Geometry check sheet. Reference: the model listing, model coordinates, mm. Face numbers are marked on the shaded views. A direction names the side the tool comes from. Coordinates: 2 decimals unless noted, no trailing zeros. Write each loop counter-clockwise with the first axis right and the second up, starting at its lowest first coordinate (ties: lowest second). Pieces come first, ordered by that corner, then holes.
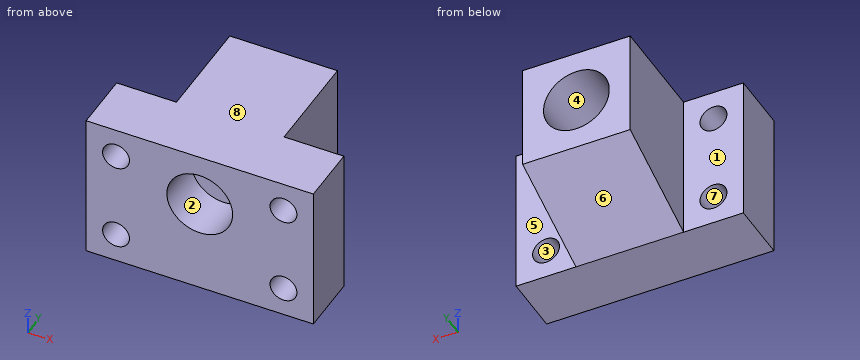
from build123d import *

# Parameters (mm, degrees)
SALIENTE_EXTRUIR1_DEPTH      = 18
SALIENTE_EXTRUIR1_DEPTH_BACK = 32
CROQUIS2_R                   = 11
CORTAR_EXTRUIR1_DEPTH        = 30
CORTAR_EXTRUIR2_START        = -16
CROQUIS3_R                   = 11
CORTAR_EXTRUIR2_DEPTH        = 16
CORTAR_EXTRUIR3_REACH        = 60.034
CROQUIS4_R                   = 5.5
CORTAR_EXTRUIR4_REACH        = 86.764
CORTAR_EXTRUIR5_REACH        = 62.77
CROQUIS6_R                   = 4.5


with BuildPart() as part:
    # Croquis1 → Saliente-Extruir1 (new, two sides: drawn at the far end of the back side and taken through both)
    with BuildSketch(Plane.XY.offset(-SALIENTE_EXTRUIR1_DEPTH_BACK)):
        Polygon((38, 0), (-38, 0), (-38, 20), (-18, 20), (-18, 55), (18, 55), (18, 20), (38, 20), align=None)
    extrude(amount=SALIENTE_EXTRUIR1_DEPTH + SALIENTE_EXTRUIR1_DEPTH_BACK)

    # Croquis2 → Cortar-Extruir1 (cut)
    with BuildSketch(Plane(origin=(0, 55, 0), x_dir=(1, 0, 0), z_dir=(0, 1, 0))):
        with Locations(Location((0, 0, 0), (0, 0, 270))):
            Circle(CROQUIS2_R)
    extrude(amount=-CORTAR_EXTRUIR1_DEPTH, mode=Mode.SUBTRACT)

    # Croquis3 → Cortar-Extruir2 (cut)
    with BuildSketch(Plane.XZ.offset(CORTAR_EXTRUIR2_START)):
        with Locations(Location((0, 0, 0), (0, 0, 90))):
            Circle(CROQUIS3_R)
    extrude(amount=CORTAR_EXTRUIR2_DEPTH, mode=Mode.SUBTRACT)

    # Croquis4 → Cortar-Extruir3 (cut, up to next)
    with BuildSketch(Plane(origin=(0, 25, 0), x_dir=(1, 0, 0), z_dir=(0, 1, 0)), mode=Mode.PRIVATE) as cortar_extruir3_sk1:
        with Locations(Location((0, 0, 0), (0, 0, 270))):
            Circle(CROQUIS4_R)
    cortar_extruir3_tool1 = extrude(cortar_extruir3_sk1.sketch, amount=-CORTAR_EXTRUIR3_REACH, mode=Mode.PRIVATE) & part.part
    add(cortar_extruir3_tool1.solids().sort_by_distance((0, 25, 0))[0], mode=Mode.SUBTRACT)

    # Croquis5 → Cortar-Extruir4 (cut, up to next)
    with BuildSketch(Plane(origin=(18, 0, 0), x_dir=(0, 0, -1), z_dir=(1, 0, 0)), mode=Mode.PRIVATE) as cortar_extruir4_sk1:
        Polygon((32, 55), (32, 20), (18, 55), align=None)
    cortar_extruir4_tool1 = extrude(cortar_extruir4_sk1.sketch, amount=-CORTAR_EXTRUIR4_REACH, mode=Mode.PRIVATE) & part.part
    add(cortar_extruir4_tool1.solids().sort_by_distance((18, 43.333333, -27.333333))[0], mode=Mode.SUBTRACT)

    # Croquis6 → Cortar-Extruir5 (cut, up to next)
    with BuildSketch(Plane(origin=(0, 20, 0), x_dir=(1, 0, 0), z_dir=(0, 1, 0)), mode=Mode.PRIVATE) as cortar_extruir5_sk1:
        with Locations(Location((-28, 22, 0), (0, 0, 270))):
            Circle(CROQUIS6_R)
    cortar_extruir5_tool1 = extrude(cortar_extruir5_sk1.sketch, amount=-CORTAR_EXTRUIR5_REACH, mode=Mode.PRIVATE) & part.part
    # Croquis6 → Cortar-Extruir5 (cut, up to next)
    with BuildSketch(Plane(origin=(0, 20, 0), x_dir=(1, 0, 0), z_dir=(0, 1, 0)), mode=Mode.PRIVATE) as cortar_extruir5_sk2:
        with Locations(Location((-28, -8, 0), (0, 0, 270))):
            Circle(CROQUIS6_R)
    cortar_extruir5_tool2 = extrude(cortar_extruir5_sk2.sketch, amount=-CORTAR_EXTRUIR5_REACH, mode=Mode.PRIVATE) & part.part
    # Croquis6 → Cortar-Extruir5 (cut, up to next)
    with BuildSketch(Plane(origin=(0, 20, 0), x_dir=(1, 0, 0), z_dir=(0, 1, 0)), mode=Mode.PRIVATE) as cortar_extruir5_sk3:
        with Locations(Location((28, 22, 0), (0, 0, 270))):
            Circle(CROQUIS6_R)
    cortar_extruir5_tool3 = extrude(cortar_extruir5_sk3.sketch, amount=-CORTAR_EXTRUIR5_REACH, mode=Mode.PRIVATE) & part.part
    # Croquis6 → Cortar-Extruir5 (cut, up to next)
    with BuildSketch(Plane(origin=(0, 20, 0), x_dir=(1, 0, 0), z_dir=(0, 1, 0)), mode=Mode.PRIVATE) as cortar_extruir5_sk4:
        with Locations(Location((28, -8, 0), (0, 0, 270))):
            Circle(CROQUIS6_R)
    cortar_extruir5_tool4 = extrude(cortar_extruir5_sk4.sketch, amount=-CORTAR_EXTRUIR5_REACH, mode=Mode.PRIVATE) & part.part
    add(cortar_extruir5_tool1.solids().sort_by_distance((-28, 20, -22))[0], mode=Mode.SUBTRACT)
    add(cortar_extruir5_tool2.solids().sort_by_distance((-28, 20, 8))[0], mode=Mode.SUBTRACT)
    add(cortar_extruir5_tool3.solids().sort_by_distance((28, 20, -22))[0], mode=Mode.SUBTRACT)
    add(cortar_extruir5_tool4.solids().sort_by_distance((28, 20, 8))[0], mode=Mode.SUBTRACT)


solid = part.part
1. Sectioned sample at A-A, the plane x = 0. Record the boundary of the cut face in (y, z), and give its area (3 significant figures).
Computed values:
outline: (0, -32) - (20, -32) - (55, -18) - (55, -11) - (25, -11) - (25, -5.5) - (16, -5.5) - (16, -11) - (0, -11) - close; (0, 11) - (16, 11) - (16, 5.5) - (25, 5.5) - (25, 11) - (55, 11) - (55, 18) - (0, 18) - close
area: 1,390 mm2
2. Thickness scan on line 1 along X through (y, z) = (13.5, -22); line 2 along Z through (x, y) = (32, 16.5); line 3 along X through (y, z) = (10, 8). Record the ranges inside material, lowest first.
Computed values:
line 1: x = -38 to -32.5, -23.5 to 23.5, 32.5 to 38
line 2: z = -32 to -24.06, -19.94 to 5.94, 10.06 to 18
line 3: x = -38 to -32.5, -23.5 to -7.55, 7.55 to 23.5, 32.5 to 38
3. Sectioned sample at C-C, the plane y = 4. Record the boundary of the cut face in (x, z).
Computed values:
outline: (-38, -32) - (38, -32) - (38, 18) - (-38, 18) - close; hole circle Ø9 at (-28, -22); hole circle Ø9 at (-28, 8); hole circle Ø22 at (0, 0); hole circle Ø9 at (28, -22); hole circle Ø9 at (28, 8)
4. Gauge pin test, flat ends, axial feed: pin 1 Ø17.5 at (y, z) = (37, -13) entering from +X; pin 2 Ø5 at (x, z) = (21.5, 7.5) entering from +Y; pin 3 Ø8 at (x, z) = (28, 8) entering from -Y; pin 4 Ø14.5 at (x, z) = (0, 0) entering from -Y. Record the tip position at first contact, or that the pin passes through.
Computed values:
pin 1: stops at x = 18
pin 2: stops at y = 20
pin 3: passes through
pin 4: stops at y = 16
5. Access from +Z, -Z, +X, -X, +Y, -Y to the whole of each face (thin tool, end or side, straight path). Record for the marked faces 1, 2, 3, 4 and 5.
Computed values:
face 1: +Z, -Z, -X, +Y
face 2: -Y
face 3: +Y, -Y
face 4: +Y
face 5: +Z, -Z, +X, +Y
6. Draft check along Z on the marked faces 6, 7 and 8. Enter one of: released by +Z, released by -Z, zero draft, split by the parting line, or undercut.
Computed values:
face 6: released by -Z
face 7: undercut
face 8: released by +Z
7. Sectioned sample at B-B, the plane z = 0. Record the boundary of the cut face in (x, y).
Computed values:
outline: (-38, 0) - (-11, 0) - (-11, 16) - (-5.5, 16) - (-5.5, 25) - (-11, 25) - (-11, 55) - (-18, 55) - (-18, 20) - (-38, 20) - close; (5.5, 16) - (11, 16) - (11, 0) - (38, 0) - (38, 20) - (18, 20) - (18, 55) - (11, 55) - (11, 25) - (5.5, 25) - close
8. Sectioned sample at D-D, the plane z = -22. Record the boundary of the cut face in (x, y).
Computed values:
outline: (-38, 0) - (-32.5, 0) - (-32.5, 20) - (-38, 20) - close; (-23.5, 0) - (23.5, 0) - (23.5, 20) - (18, 20) - (18, 45) - (-18, 45) - (-18, 20) - (-23.5, 20) - close; (32.5, 0) - (38, 0) - (38, 20) - (32.5, 20) - close
